from build123d import *

# Parameters (mm, degrees)
SKETCH_1_R          = 18.5
EXTRUDE_1_DEPTH     = 46
SKETCH_1_3_R        = 1.5
CUT_EXTRUDE_1_DEPTH = 6
SKETCH_2_R          = 6
EXTRUDE_2_DEPTH     = 6
SKETCH_3_R          = 3
EXTRUDE_3_DEPTH     = 15.5
SKETCH_5_R          = 18.5
EXTRUDE_4_DEPTH     = 11.5


with BuildPart() as part:
    # Sketch 1 → Extrude 1 (new body)
    with BuildSketch(Plane.XY):
        Circle(SKETCH_1_R)
    extrude(amount=EXTRUDE_1_DEPTH)

    # Sketch 1_3 → Cut-Extrude 1 (cut)
    with BuildSketch(Plane.XY):
        with Locations((7.272414017, -13.688023757)):
            Circle(SKETCH_1_3_R)
        with Locations((-8.217969292, -13.142107164)):
            Circle(SKETCH_1_3_R)
        with Locations((-15.490383309, 0.545916592)):
            Circle(SKETCH_1_3_R)
        with Locations((8.217969292, 13.142107164)):
            Circle(SKETCH_1_3_R)
        with Locations((-7.272414017, 13.688023757)):
            Circle(SKETCH_1_3_R)
        with Locations((15.490383309, -0.545916592)):
            Circle(SKETCH_1_3_R)
    extrude(amount=CUT_EXTRUDE_1_DEPTH, mode=Mode.SUBTRACT)

    # Sketch 2 → Extrude 2 (add)
    with BuildSketch(Plane(origin=(0, 0, 0), x_dir=(-1, 0, 0), z_dir=(0, 0, -1))):
        with Locations(Location((-0.246542977, 6.995656978, 0), (0, 0, 180))):
            Circle(SKETCH_2_R)
    extrude(amount=EXTRUDE_2_DEPTH)

    # Sketch 3 → Extrude 3 (add)
    with BuildSketch(Plane(origin=(0, 0, -6), x_dir=(-1, 0, 0), z_dir=(0, 0, -1))):
        with Locations((-0.246542977, 6.995656978)):
            Circle(SKETCH_3_R)
    extrude(amount=EXTRUDE_3_DEPTH)

    # Sketch 5 → Extrude 4 (add)
    with BuildSketch(Plane.XY.offset(46)):
        Circle(SKETCH_5_R)
    extrude(amount=EXTRUDE_4_DEPTH)


solid = part.part
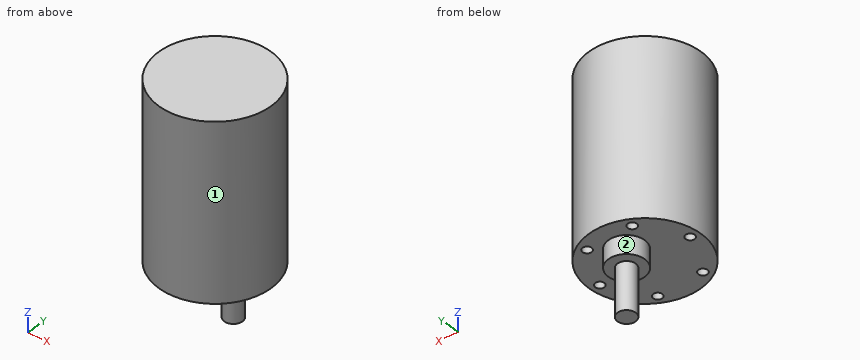
Design review of the part built by this model. Coordinates are the model's own, in mm. Face numbers are marked on the shaded views. A direction names the side the tool comes from. Coordinates: 2 decimals unless noted, no trailing zeros. Write each loop counter-clockwise with the first axis right and the second up, starting at its lowest first coordinate (ties: lowest second). Pieces come first, ordered by that corner, then holes. Notation, with made-up numbers: (28.25, 1) -> (52.25, 1) arc R35 cw to (52.25, 40) -> close; hole circle Ø4 at (50.5, -8.75). An arc over 180 degrees is marked (long way). Write each question's results on one line, items separated by ' | '. Start each with the question number.
(1) For line 1 along X through (y, z) = (-12.5, 4.5); line 2 along Z through (x, y) = (14.5, -5.5); line 3 along Z through (x, y) = (-5, 5), list the stretches that pass through material, from the lowest coordinate up. Write a range as from..to.
(2) Clearance check with flat-ended pins moving along their axes: P1, Ø2, axis at x = -12.5, z = 25, coming from the +Y side; P2, Ø0.9, axis at x = -7.5, y = 14, coming from the -Z side; P3, Ø12, axis at x = 5.5, z = -13, coming from the -Y side; P4, Ø4, axis at y = 1.5, z = -10, coming from the -X side. State where each tip first meets the part, or that it passes through.
(3) Tool access review of the marked faces 1 and 2: name each direction out of +Z, -Z, +X, -X, +Y, -Y from which nothing blocks a thin tool from reaching the whole face with its end or side.
(4) Take a section at B-B on y = 8.5. Write out the cut boundary in (x, z), and give its area (3 significant figures).
(5) Take a section at A-A on z = 5. Write out the cut boundary in (x, y), and give its area (3 significant figures).
(6) Take a section at C-C on z = 20. Write out the cut boundary in (x, y).
(7) Take a section at D-D on x = 0. Write out the cut boundary in (y, z), and give its area (3 significant figures).
Results found:
1) line 1: x = -13.64..-9.57, -6.86..6.36, 8.19..13.64 | line 2: z = 0..57.5 | line 3: z = -6..57.5
2) P1: stops at y = 14.49 | P2: stops at z = 6 | P3: stops at y = 4 | P4: passes through
3) face 1: +Z, -Z | face 2: -Z
4) outline: (-16.43, 0) -> (-5.56, 0) -> (-5.56, -6) -> (-2.35, -6) -> (-2.35, -21.5) -> (2.84, -21.5) -> (2.84, -6) -> (6.05, -6) -> (6.05, 0) -> (16.43, 0) -> (16.43, 57.5) -> (-16.43, 57.5) -> close | area: 2,040 mm2
5) outline: circle Ø37 at (0, 0); hole circle Ø3 at (-15.49, 0.55); hole circle Ø3 at (-8.22, -13.14); hole circle Ø3 at (-7.27, 13.69); hole circle Ø3 at (7.27, -13.69); hole circle Ø3 at (8.22, 13.14); hole circle Ø3 at (15.49, -0.55) | area: 1,030 mm2
6) outline: circle Ø37 at (0, 0)
7) outline: (-18.5, 0) -> (1, 0) -> (1, -6) -> (4.01, -6) -> (4.01, -21.5) -> (9.99, -21.5) -> (9.99, -6) -> (12.99, -6) -> (12.99, 0) -> (18.5, 0) -> (18.5, 57.5) -> (-18.5, 57.5) -> close | area: 2,290 mm2
